Geometry: see drawing. Coordinates: mm, zero at the bounding-box minimum. A direction names the side the tool comes from. Round coordinates to 2 decimals unless told otherwise and drop trailing zeros. Order: outer loops, then holes, each group sorted by start corner. A loop starts at its lowest first (then second) coordinate and runs counter-clockwise, first axis right, second up. Notation, with made-up numbers: (47, 34.5) -> (106, 34.5) arc R26 cw to (106, 64.5) -> close; hole circle Ø6 at (-16, 20). An arc over 180 degrees is marked (long way). One line per item, written item: value. Start each with the question number.
1) Section B-B (y = 40). Return the cut outline in (x, z), and give its area (3 significant figures).
2) Section A-A (x = 38.75). Return the cut outline in (y, z).
3) Pin query (flat end, axial travel): P1, Ø6.5, axis at x = 30.75, z = 42, coming from the +Y side; P2, Ø8, axis at x = 16.5, z = 25.5, coming from the -Y side; P3, Ø8, axis at y = 48, z = 39, coming from the -X side; P4, Ø5, axis at y = 22.5, z = 8.5, coming from the -X side. Return the tip coordinate at first contact, or that it passes through.
4) Ray query, L1, parallel to X at y = 53.8, z = 42; L2, parallel to Z at x = 14, y = 54; L3, parallel to X at y = 53, z = 18. Return the intervals inside material, ascending.
5) Section C-C (z = 25). State how many separate pieces and enclosed holes the cut face has, and give its area (3 significant figures).
6) Section D-D (x = 14.75). Return the cut outline in (y, z).
7) Reachability of the marked faces 1 and 2 from +Z, -Z, +X, -X, +Y, -Y: full face, straight path, thin tool, end or side. Return the list, or none.
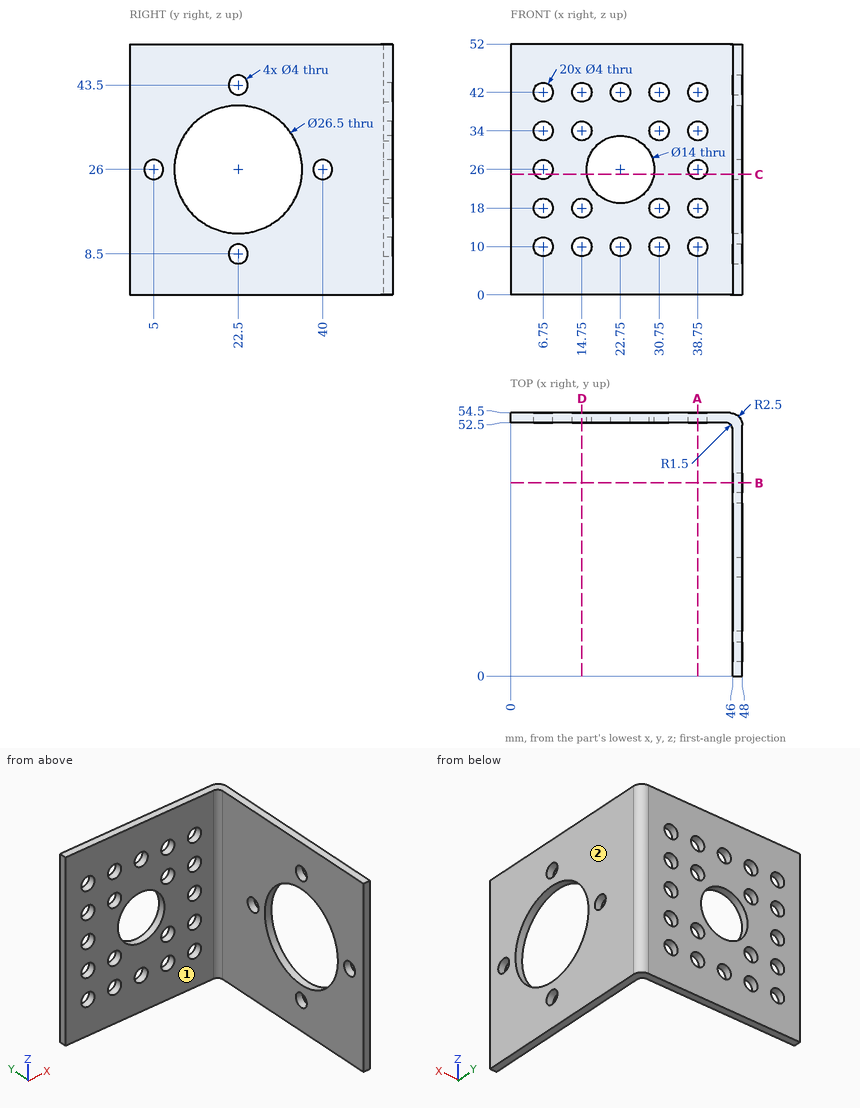
Findings:
1. outline: (46, 0) -> (48, 0) -> (48, 24) -> (46, 24) -> close; (46, 28) -> (48, 28) -> (48, 52) -> (46, 52) -> close
1. area: 96.0 mm2
2. outline: (52.5, 0) -> (54.5, 0) -> (54.5, 8) -> (52.5, 8) -> close; (52.5, 12) -> (54.5, 12) -> (54.5, 16) -> (52.5, 16) -> close; (52.5, 20) -> (54.5, 20) -> (54.5, 24) -> (52.5, 24) -> close; (52.5, 28) -> (54.5, 28) -> (54.5, 32) -> (52.5, 32) -> close; (52.5, 36) -> (54.5, 36) -> (54.5, 40) -> (52.5, 40) -> close; (52.5, 44) -> (54.5, 44) -> (54.5, 52) -> (52.5, 52) -> close
3. P1: y = 54.5
3. P2: y = 52.5
3. P3: x = 45.62
3. P4: x = 46
4. L1: 0 to 4.75, 8.75 to 12.75, 16.75 to 20.75, 24.75 to 28.75, 32.75 to 36.75, 40.75 to 47.23
4. L2: 0 to 8.15, 11.85 to 16.15, 19.85 to 32.15, 35.85 to 40.15, 43.85 to 52
4. L3: 0 to 4.75, 8.75 to 12.75, 16.75 to 28.75, 32.75 to 36.75, 40.75 to 47.79
5. separate pieces: 7
5. enclosed holes: 0
5. area: 91.9 mm2
6. outline: (52.5, 0) -> (54.5, 0) -> (54.5, 8) -> (52.5, 8) -> close; (52.5, 12) -> (54.5, 12) -> (54.5, 16) -> (52.5, 16) -> close; (52.5, 20) -> (54.5, 20) -> (54.5, 32) -> (52.5, 32) -> close; (52.5, 36) -> (54.5, 36) -> (54.5, 40) -> (52.5, 40) -> close; (52.5, 44) -> (54.5, 44) -> (54.5, 52) -> (52.5, 52) -> close
7. face 1: +Z, -Z, -X, -Y
7. face 2: +Z, -Z, +X, +Y, -Y
